from build123d import *

# Parameters (mm, degrees)
BOSS_EXTRUDE1_DEPTH      = 5
BOSS_EXTRUDE1_DEPTH_BACK = 5
CIRPATTERN1_COUNT        = 3
SKETCH7_R                = 1.725
CUT_EXTRUDE2_DEPTH       = 47.868710659
CIRPATTERN2_COUNT        = 3
CUT_EXTRUDE3_DEPTH       = 47.751214304
CUT_EXTRUDE3_DEPTH_BACK  = 47.751214304
SKETCH8_R                = 8.5
SKETCH8_R_2              = 1.625
SKETCH9_R                = 8.5
SKETCH9_R_2              = 6.75
BOSS_EXTRUDE2_DEPTH      = 6.3


with BuildPart() as part:
    # Sketch4 → Boss-Extrude1 (new, two sides: drawn at the far end of the back side and taken through both)
    with BuildSketch(Plane(origin=(0, 0, 0), x_dir=(1, 0, 0), z_dir=(0, 1, 0)).offset(-BOSS_EXTRUDE1_DEPTH_BACK)):
        with BuildLine():
            Line((23.846787517, 20.696152423), (13.522711642, 14.735544437))
            ThreePointArc((13.522711642, 14.735544437), (17.320508076, 10), (19.522711642, 4.343239591))
            Line((19.522711642, 4.343239591), (29.846787517, 10.303847577))
            Line((29.846787517, 10.303847577), (34.346787517, 2.509618943))
            Line((34.346787517, 2.509618943), (23.954482672, -3.490381057))
            Line((23.954482672, -3.490381057), (15, -19))
            Line((15, -19), (15, -31))
            Line((15, -31), (6, -31))
            Line((6, -31), (6, -19.078784028))
            ThreePointArc((6, -19.078784028), (0, -20), (-6, -19.078784028))
            Line((-6, -19.078784028), (-6, -31))
            Line((-6, -31), (-15, -31))
            Line((-15, -31), (-15, -19))
            Line((-15, -19), (-23.954482672, -3.490381057))
            Line((-23.954482672, -3.490381057), (-34.346787517, 2.509618943))
            Line((-34.346787517, 2.509618943), (-29.846787517, 10.303847577))
            Line((-29.846787517, 10.303847577), (-19.522711642, 4.343239591))
            ThreePointArc((-19.522711642, 4.343239591), (-17.320508076, 10), (-13.522711642, 14.735544437))
            Line((-13.522711642, 14.735544437), (-23.846787517, 20.696152423))
            Line((-23.846787517, 20.696152423), (-19.346787517, 28.490381057))
            Line((-19.346787517, 28.490381057), (-8.954482672, 22.490381057))
            Line((-8.954482672, 22.490381057), (8.954482672, 22.490381057))
            Line((8.954482672, 22.490381057), (19.346787517, 28.490381057))
            Line((19.346787517, 28.490381057), (23.846787517, 20.696152423))
        make_face()
    extrude(amount=BOSS_EXTRUDE1_DEPTH + BOSS_EXTRUDE1_DEPTH_BACK)

    # Sketch6 → Revolve1 (revolve)
    with BuildSketch(Plane(origin=(0, 0, 0), x_dir=(1, 0, 0), z_dir=(0, 1, 0))):
        Polygon((-15, -25), (-20, -25), (-20, -28), (-15, -31), align=None)
        Polygon((15, -31), (15, -25), (20, -25), (20, -28), align=None)
    revolve1 = revolve(axis=Axis((-15, 0, 25), (1, 0, 0)))

    # CirPattern1: Revolve1 ×3 about axis
    cirpattern1_axis = Axis((0, 0, 0), (0, 1, 0))
    for i in range(1, CIRPATTERN1_COUNT):
        add(revolve1.rotate(cirpattern1_axis, i * 360 / CIRPATTERN1_COUNT))

    # Sketch7 → Cut-Extrude2 (cut, symmetric)
    with BuildSketch(Plane(origin=(0, 0, 0), x_dir=(0, 0, -1), z_dir=(1, 0, 0))):
        with Locations((-25, 0)):
            Circle(SKETCH7_R)
        with BuildLine():
            Line((-28.31662479, 5), (-19, 5))
            Line((-19, 5), (-19, 25))
            Line((-19, 25), (-39, 25))
            Line((-39, 25), (-39, -25))
            Line((-39, -25), (-19, -25))
            Line((-19, -25), (-19, -5))
            Line((-19, -5), (-28.31662479, -5))
            ThreePointArc((-28.31662479, -5), (-31, 0), (-28.31662479, 5))
        make_face()
    cut_extrude2 = extrude(amount=CUT_EXTRUDE2_DEPTH, both=True, mode=Mode.SUBTRACT)

    # CirPattern2: Cut-Extrude2 ×3 about axis
    cirpattern2_axis = Axis((0, 5, 0), (0, 1, 0))
    for i in range(1, CIRPATTERN2_COUNT):
        add(cut_extrude2.rotate(cirpattern2_axis, i * 360 / CIRPATTERN2_COUNT), mode=Mode.SUBTRACT)

    # Sketch8 → Cut-Extrude3 (cut, two sides: drawn at the far end of the back side and taken through both)
    with BuildSketch(Plane(origin=(0, 0, 0), x_dir=(1, 0, 0), z_dir=(0, 1, 0)).offset(-CUT_EXTRUDE3_DEPTH_BACK)):
        with Locations(Location((0, 0, 0), (0, 0, 270))):
            Circle(SKETCH8_R)
        with Locations(Location((-12.5, 0, 0), (0, 0, 270))):
            Circle(SKETCH8_R_2)
        with Locations(Location((-6.25, 10.825317547, 0), (0, 0, 270))):
            Circle(SKETCH8_R_2)
        with Locations(Location((6.25, 10.825317547, 0), (0, 0, 270))):
            Circle(SKETCH8_R_2)
        with Locations(Location((12.5, 0, 0), (0, 0, 270))):
            Circle(SKETCH8_R_2)
        with Locations(Location((6.25, -10.825317547, 0), (0, 0, 270))):
            Circle(SKETCH8_R_2)
        with Locations(Location((-6.25, -10.825317547, 0), (0, 0, 270))):
            Circle(SKETCH8_R_2)
    extrude(amount=CUT_EXTRUDE3_DEPTH + CUT_EXTRUDE3_DEPTH_BACK, mode=Mode.SUBTRACT)

    # Sketch9 → Boss-Extrude2 (add)
    with BuildSketch(Plane(origin=(0, 5, 0), x_dir=(1, 0, 0), z_dir=(0, 1, 0))):
        with Locations(Location((0, 0, 0), (0, 0, 270))):
            Circle(SKETCH9_R)
        with Locations(Location((0, 0, 0), (0, 0, 270))):
            Circle(SKETCH9_R_2, mode=Mode.SUBTRACT)
    extrude(amount=-BOSS_EXTRUDE2_DEPTH)


solid = part.part
Design review of the part built by this model. Coordinates are the model's own, in mm. A direction names the side the tool comes from. Round coordinates to 2 decimals unless told otherwise and drop trailing zeros. Write each loop counter-clockwise with the first axis right and the second up, starting at its lowest first coordinate (ties: lowest second). Pieces come first, ordered by that corner, then holes. Notation, with made-up numbers: M 40,-7.75 L 93,-7.75 A19 ccw 93,9.25 Z; hole C 73.25,23.25 d11. An arc over 180 degrees is marked long. One line per item, written item: value. Start each with the question number.
1. Take a section at A-A on x = 0. State the section outline as (y, z) points, then the cut area to 3 significant figures.
2. Clearance check with flat-ended pins moving along their axes: P1, Ø4, axis at x = 27, y = 0.5, coming from the -Z side; P2, Ø1.5, axis at y = 1, z = -15, coming from the +X side; P3, Ø4.5, axis at y = 0, z = 25, coming from the -X side. State where each tip first meets the part, or that it passes through.
3. Draft analysis for pull direction X (two halves, no side actions). For faces 6 (the face through (29.955, -0.042, 5.8)), 7 (the face through (-5.762, -0.07, 12.375)), 8 (the face through (-18.612, -2.292, -17.674)), state which applies: pulls with the +X half, pulls with the -X half, needs draft (parallel to the pull), parting line crosses it, or undercut.
4. Take a section at B-B on z = 25. State the section outline as (x, y) points (3 decimals), then the cut area to 3 significant figures.
5. To check wall thickness, follow probe 1 along X at (y, z) = (0, 27); probe 2 along Z at (x, y) = (-16.5, 3.5); probe 3 along Z at (x, y) = (12.75, 0) (3 decimals). State the ranges of each line that lie inside material, in increasing order. Write a range as from..to.
6. For faces 1 (the face through (9.68, -3.81, -22.91)), 2 (the face through (-24.595, 3.785, 3.121)), 3 (the face through (8, 5, 0)), 4 (the face through (-9.519, 3.785, -22.817)), 5 (the face through (19.54, -0.07, 11.14)), list the 3-axis set-ups (+Z, -Z, +X, -X, +Y, -Y) from which the entire face can be reached by the end or side of a thin tool; tool diameter is ignored.
7. Take a section at C-C on x = -12.5. State how many separate pieces and enclosed holes the cut face has, then the cut area to 3 significant figures.
Computed:
1. outline: M -5,-22.49 L 5,-22.49 L 5,-6.75 L -1.3,-6.75 L -1.3,-8.5 L -5,-8.5 Z; M -5,8.5 L -1.3,8.5 L -1.3,6.75 L 5,6.75 L 5,20 L -5,20 Z
1. area: 277 mm²
2. P1: stops at z = -9.81
2. P2: stops at x = 15.28
2. P3: stops at x = -20
3. face 6: pulls with the +X half
3. face 7: undercut
3. face 8: pulls with the -X half
4. outline: M -20,-3 L -16.667,-5 L -6,-5 L -6,-1.725 L -20,-1.725 Z; M -20,1.725 L -6,1.725 L -6,5 L -16.667,5 L -20,3 Z; M 6,-5 L 16.667,-5 L 20,-3 L 20,-1.725 L 6,-1.725 Z; M 6,1.725 L 20,1.725 L 20,3 L 16.667,5 L 6,5 Z
4. area: 170 mm²
5. probe 1: x = -20..-6, 6..20
5. probe 2: z = -28.69..-16.45, -11.3..16.4, 21.29..28.71
5. probe 3: z = -24.466..-1.606, 1.606..23.275, 26.725..31
6. face 1: -Z, -Y
6. face 2: +Z, +Y
6. face 3: +Z, -Z, +X, -X, +Y
6. face 4: -Z, +Y
6. face 5: +Y, -Y
7. separate pieces: 2
7. enclosed holes: 1
7. area: 540 mm²
